CAD build for the part. Positions are in the model's coordinates, mm. Coordinates: 2 decimals unless noted, no trailing zeros. Order: outer loops, then holes, each group sorted by start corner. A loop starts at its lowest first (then second) coordinate and runs counter-clockwise, first axis right, second up.
from build123d import *

# Parameters (mm, degrees)
CROQUIS3_R                                           = 3.175
SALIENTE_EXTRUIR2_DEPTH                              = 10.922
REFRENTADO_PARA_TORNILLO_CON_CABEZA_HUEC_D           = 3.048
REFRENTADO_PARA_TORNILLO_CON_CABEZA_HUEC_CBORE_D     = 4.699
REFRENTADO_PARA_TORNILLO_CON_CABEZA_HUEC_CBORE_DEPTH = 17.145
CHAFL_N1_SIZE                                        = 2.413
CHAFL_N1_SIZE2                                       = 1.22948491


with BuildPart() as part:
    # Croquis3 → Saliente-Extruir2 (new, symmetric)
    with BuildSketch(Plane.XY):
        Circle(CROQUIS3_R)
    extrude(amount=SALIENTE_EXTRUIR2_DEPTH, both=True)

    # Refrentado para tornillo con cabeza hueca de 1/41 (through all)
    with Locations(Plane(origin=(0, 0, -10.922), x_dir=(-1, 0, 0), z_dir=(0, 0, -1))):
        with Locations((0, 0)):
            CounterBoreHole(REFRENTADO_PARA_TORNILLO_CON_CABEZA_HUEC_D / 2, REFRENTADO_PARA_TORNILLO_CON_CABEZA_HUEC_CBORE_D / 2, REFRENTADO_PARA_TORNILLO_CON_CABEZA_HUEC_CBORE_DEPTH)

    # Chaflán1
    chafl_n1_edges = [part.edges().sort_by_distance(p)[0] for p in [
        (-3.175, 0, 10.922),
    ]]
    chafl_n1_side = [part.faces().sort_by_distance(p)[0] for p in [
        (-3.175, 0, 0),
    ]]
    chamfer(chafl_n1_edges, length=CHAFL_N1_SIZE, length2=CHAFL_N1_SIZE2, reference=chafl_n1_side[0])


solid = part.part
1) Two-plate mould, pull along Y, no slides. Class faces 1 (the cylindrical face through (-0.69, -3.1, -1.07)), 2 (the cylindrical face through (-0.2, 1.51, 8.61)): released by +Y, released by -Y, zero draft, split by the parting line, or undercut.
2) Pin check, flat tips, straight feed: P1, Ø2, axis at x = -2, z = -6.5, coming from the +Y side; P2, Ø3, axis at x = 1, y = -0.5, coming from the +Z side; P3, Ø1.5, axis at y = -2.5, z = 7.5, coming from the +X side; P4, Ø2, axis at x = 1.5, z = 5, coming from the +Y side. Stop position of each tip, or through.
3) Slice it at C-C (z = 7.5). List the corners of the cut face in (x, y) (3 decimals), plus the area to 3 significant figures.
4) Slice it at A-A (x = 0). List the corners of the cut face in (y, z) (1 decimal), plus the area to 3 significant figures.
5) Drill centre lines: probe 1 along Y at (x, z) = (0, 7.9) (3 decimals); probe 2 along Z at (x, y) = (-0.25, -1.75); probe 3 along Y at (x, z) = (1, -7.75). Where is each one in solid material? Low to high.
Worked out:
1. face 1: split by the parting line
1. face 2: undercut
2. P1: stops at y = 3.01
2. P2: stops at z = 10.92
2. P3: stops at x = 2.65
2. P4: stops at y = 3.14
3. outline: circle Ø6.35 at (0, 0); hole circle Ø3.048 at (0, 0)
3. area: 24.4 mm2
4. outline: (-3.2, -10.9) - (-2.3, -10.9) - (-2.3, 6.2) - (-1.5, 6.2) - (-1.5, 10.9) - (-1.9, 10.9) - (-3.2, 8.5) - close; (1.5, 6.2) - (2.3, 6.2) - (2.3, -10.9) - (3.2, -10.9) - (3.2, 8.5) - (1.9, 10.9) - (1.5, 10.9) - close
4. area: 40.9 mm2
5. probe 1: y = -3.175 to -1.524, 1.524 to 3.175
5. probe 2: z = 6.22 to 10.92
5. probe 3: y = -3.01 to -2.13, 2.13 to 3.01
